Check sheet for the modelled part. Datum: model origin and axes. Units: mm. A direction names the side the tool comes from. Round coordinates to 2 decimals unless told otherwise and drop trailing zeros. Write each loop counter-clockwise with the first axis right and the second up, starting at its lowest first coordinate (ties: lowest second). Pieces come first, ordered by that corner, then holes.
Item 1: Cross-section at A-A on y = 0. Enter the section's corners in (x, z).
Item 2: Cross-section at C-C on z = 32.5. Enter the section's corners in (x, y), plus the area to 3 significant figures.
Item 3: Release check for a two-part mould opening along Y. For faces 1 (the flat face through (0, 0, 10)), 2 (the cylindrical face through (9.443, 2.974, 5.423)), 3 (the flat face through (0, 0, 41)) record: +Y half, -Y half, draft (parallel to the pull), parting line (faces both ways), or undercut.
Item 4: Go/stop test with flat-tipped pins: pin 1 Ø4.5 at (x, y) = (-1.5, 1) entering from -Z; pin 2 Ø10 at (x, z) = (-6.5, 20.5) entering from +Y; pin 3 Ø5 at (y, z) = (4, 30.5) entering from -X. Record where each tip stops, or that it passes through.
Item 5: Material ranges on line 1 (Y direction, x = 0, z = 6); line 2 (Y direction, x = -0.25, z = 14); line 3 (Z direction, x = 7.25, y = -1.5), recorded low to high.
Item 6: Cross-section at D-D on y = 2.5. Enter the section's corners in (x, z).
Item 7: Tool access check on faces 4 (the cylindrical face through (0, -2, 30)), 5 (the flat face through (-7, -4, 0)), 6 (the cylindrical face through (-6.269, -4.807, 4.93)). Record the directions out of +Z, -Z, +X, -X, +Y, -Y that give a thin tool (end or side, any length) a straight path to the whole face; none if there is none.
from build123d import *

# Parameters (mm, degrees)
CROQUIS1_R              = 9.9
CROQUIS1_R_2            = 7.9
SALIENTE_EXTRUIR1_DEPTH = 10
CROQUIS2_R              = 9.9
SALIENTE_EXTRUIR2_DEPTH = 1
CROQUIS4_R              = 5
SALIENTE_EXTRUIR4_DEPTH = 9
CROQUIS3_R              = 2
SALIENTE_EXTRUIR3_DEPTH = 30


with BuildPart() as part:
    # Croquis1 → Saliente-Extruir1 (new body)
    with BuildSketch(Plane.XY):
        Circle(CROQUIS1_R)
        Circle(CROQUIS1_R_2, mode=Mode.SUBTRACT)
    extrude(amount=SALIENTE_EXTRUIR1_DEPTH)

    # Croquis2 → Saliente-Extruir2 (add)
    with BuildSketch(Plane.XY.offset(10)):
        Circle(CROQUIS2_R)
    extrude(amount=SALIENTE_EXTRUIR2_DEPTH)

    # Croquis4 → Saliente-Extruir4 (add)
    with BuildSketch(Plane.XY.offset(11)):
        Circle(CROQUIS4_R)
    extrude(amount=SALIENTE_EXTRUIR4_DEPTH)

    # Croquis3 → Saliente-Extruir3 (add)
    with BuildSketch(Plane.XY.offset(11)):
        Circle(CROQUIS3_R)
    extrude(amount=SALIENTE_EXTRUIR3_DEPTH)


solid = part.part
Response values:
1. outline: (-9.9, 0) - (-7.9, 0) - (-7.9, 10) - (7.9, 10) - (7.9, 0) - (9.9, 0) - (9.9, 11) - (5, 11) - (5, 20) - (2, 20) - (2, 41) - (-2, 41) - (-2, 20) - (-5, 20) - (-5, 11) - (-9.9, 11) - close
2. outline: circle Ø4 at (0, 0)
2. area: 12.6 mm2
3. face 1: undercut
3. face 2: parting line
3. face 3: draft
4. pin 1: stops at z = 10
4. pin 2: stops at y = 4.76
4. pin 3: stops at x = -1.32
5. line 1: y = -9.9 to -7.9, 7.9 to 9.9
5. line 2: y = -4.99 to 4.99
5. line 3: z = 10 to 11
6. outline: (-9.58, 0) - (-7.49, 0) - (-7.49, 10) - (7.49, 10) - (7.49, 0) - (9.58, 0) - (9.58, 11) - (4.33, 11) - (4.33, 20) - (-4.33, 20) - (-4.33, 11) - (-9.58, 11) - close
7. face 4: +Z
7. face 5: -Z, +X, -X, +Y, -Y
7. face 6: -Z
